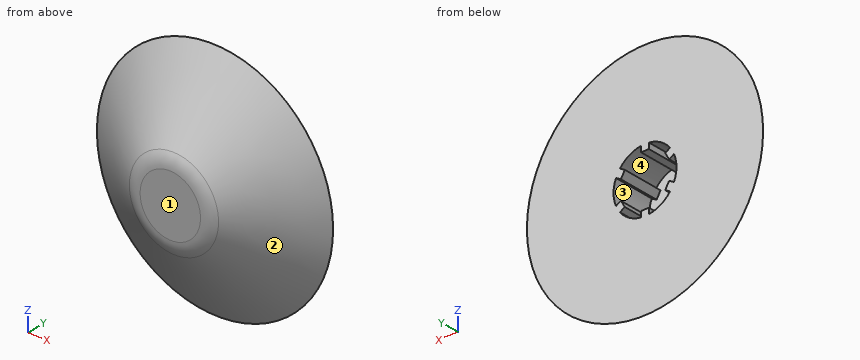
Autodesk Fusion 360 part; units mm, degrees
sketch "Sketch1" plane through (0, 0, 0) normal (0, 1, 0) x (1, 0, 0)
  circle A0 centre (0, 0) radius 5.25
  circle A1 centre (0, 0) radius 7.25
  dimension "d1" = 10.5
  dimension "d2" = 2
extrude "Extrude1" add sketch "Sketch1" along normal blind 6
sketch "Sketch2" plane through (0, 0, 0) normal (0, -1, 0) x (1, 0, 0)
  circle A0 centre (0, 0) radius 5.25
  circle A1 centre (0, 0) radius 7.25
  circle A2 centre (0, 0) radius 7.25
extrude "Extrude2" add sketch "Sketch2" along normal blind 4 contours A0 | A1 A2
sketch "Sketch3" plane through (0, 6, 0) normal (0, 1, 0) x (-1, 0, 0)
  circle A0 centre (0, 0) radius 5.25
  circle A1 centre (0, 0) radius 7.25
  circle A2 centre (0, 0) radius 7.25
  circle A3 centre (0, 0) radius 22.5
  dimension "d7" = 45
loft "Loft1" add profiles "Sketch3" section 1 contours A3 section 2 face at (1.965, -4, -0.3602)
sketch "Sketch4" plane through (0, 6, 0) normal (0, 1, 0) x (-1, 0, 0)
  circle A0 centre (0, 0) radius 22.5
  circle A1 centre (0, 0) radius 4.875 construction
  circle A2 centre (0, 0) radius 6
  line L0 (0, 0) -> (0, -6) construction
  line L1 (-0.75, -6) -> (0.75, -6)
  line L2 (0.75, -6) -> (0.75, -4.875)
  line L3 (0.75, -4.875) -> (-0.75, -4.875)
  line L4 (-0.75, -4.875) -> (-0.75, -6)
  line L5 (-0.75, -6) -> (0.75, -4.875) construction
  line L6 (0.75, -6) -> (-0.75, -4.875) construction
  line L7 (5.5712, -2.3505) -> (4.5969, -1.788)
  line L8 (4.5969, -1.788) -> (3.8469, -3.087)
  line L9 (3.8469, -3.087) -> (4.8212, -3.6495)
  line L10 (4.8212, -3.6495) -> (5.5712, -2.3505)
  line L11 (4.8212, 3.6495) -> (3.8469, 3.087)
  line L12 (3.8469, 3.087) -> (4.5969, 1.788)
  line L13 (4.5969, 1.788) -> (5.5712, 2.3505)
  line L14 (5.5712, 2.3505) -> (4.8212, 3.6495)
  line L15 (-0.75, 6) -> (-0.75, 4.875)
  line L16 (-0.75, 4.875) -> (0.75, 4.875)
  line L17 (0.75, 4.875) -> (0.75, 6)
  line L18 (0.75, 6) -> (-0.75, 6)
  line L19 (-5.5712, 2.3505) -> (-4.5969, 1.788)
  line L20 (-4.5969, 1.788) -> (-3.8469, 3.087)
  line L21 (-3.8469, 3.087) -> (-4.8212, 3.6495)
  line L22 (-4.8212, 3.6495) -> (-5.5712, 2.3505)
  line L23 (-4.8212, -3.6495) -> (-3.8469, -3.087)
  line L24 (-3.8469, -3.087) -> (-4.5969, -1.788)
  line L25 (-4.5969, -1.788) -> (-5.5712, -2.3505)
  line L26 (-5.5712, -2.3505) -> (-4.8212, -3.6495)
  point P0 (0, -5.4375)
  dimension "d8" = 9.75
  dimension "d9" = 12
  dimension "d10" = 1.5
  dimension "d12" = 360
extrude "Extrude3" cut sketch "Sketch4" against normal blind 8 contours A2 L2 L3 L4 L7 L8 L9 L11 L12 L13 L15 L16 L17 L19 L20 L21 L23 L24 L25
fillet "Fillet1" radius 5 1 edges at (-6.7594, -4, -2.6217)
Design review of the part built by this model. Coordinates are the model's own, in mm. Face numbers are marked on the shaded views. Round coordinates to 2 decimals unless told otherwise and drop trailing zeros. Order: outer loops, then holes, each group sorted by start corner. A loop starts at its lowest first (then second) coordinate and runs counter-clockwise, first axis right, second up. Notation, with made-up numbers: M 57.25,-1 L 75.25,-1 A16 ccw 75.25,29 Z; hole C 18.5,49 d10. An arc over 180 degrees is marked long. Put each result on its own line as item: value.
Q1. To check wall thickness, follow line 1 (Z direction, x = 4, y = -0.5); line 2 (Z direction, x = 1, y = -0.5); line 3 (Y direction, x = -6.5, z = -5.5). State the ranges of each line that lie inside material, in increasing order.
Reported:
line 1: -11.94 to -4.47, -3.18 to -2.82, 2.82 to 3.18, 4.47 to 11.94
line 2: -12.55 to -5.92, 5.92 to 12.55
line 3: -3.17 to 6
Q2. Consider section B-B (x = 0). State the section outline as (y, z) points (3 decimals).
Reported:
outline: M -4,-5.757 A5 ccw -3.181,-8.499 L 6,-22.5 L 6,-4.875 L -2,-4.875 L -2,4.875 L 6,4.875 L 6,22.5 L -3.181,8.499 A5 ccw -4,5.757 Z
Q3. Draft analysis for pull direction X (two halves, no side actions). For the marked faces 1, 2, 3 and 4, state which applies: released by +X, released by -X, zero draft, split by the parting line, or undercut.
Reported:
face 1: zero draft
face 2: split by the parting line
face 3: undercut
face 4: undercut
Q4. Insertion check: pin 1 Ø0.5 at (y, z) = (3, -5.5) entering from +X; pin 2 Ø1 at (y, z) = (0.5, 6) entering from -X; pin 3 Ø1.2 at (y, z) = (1.5, 5.5) entering from +X. Each pin has a flat end and moves straight along its axis. Give the tip position at first contact, or say it passes through.
Reported:
pin 1: x = 17.47
pin 2: x = -13.64
pin 3: x = 15.63
